Could you check a few things on this model? Use its own coordinates, in mm. Face numbers are marked on the shaded views. Give positions to 0.01 mm unless a question says otherwise; leave off trailing zeros. Put each result on its own line as item: value.
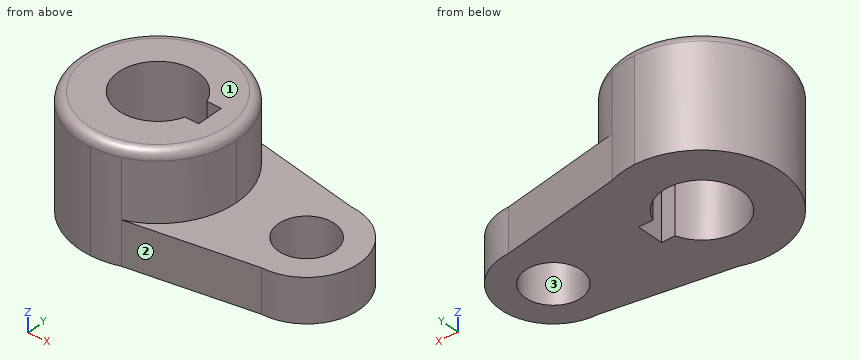
from build123d import *

# Parameters (mm, degrees)
F0_R     = 14.2875
F1_DEPTH = 40.2336
F0_R_2   = 10.16
F2_DEPTH = 15.7734
F4_DEPTH = 40.2336


# Not quite as in the source:
# - a fillet or chamfer that OpenCascade refuses, or shapes differently, is made with other operations: its cross-section is extruded or revolved along the edge and cut away or added


with BuildPart() as f1:
    # F0 (on Top) → F1 (new body)
    with BuildSketch(Plane.XY):
        with BuildLine():
            ThreePointArc((9.780704698, 26.8489932886), (4.9659159165, 28.1401901932), (0, 28.575))
            Line((0, 28.575), (9.780704698, 26.8489932886))
        make_face()
        with BuildLine():
            Line((9.780704698, -26.8489932886), (0, -28.575))
            ThreePointArc((0, -28.575), (4.9659159165, -28.1401901932), (9.780704698, -26.8489932886))
        make_face()
        with BuildLine():
            Line((9.780704698, 26.8489932886), (0, 28.575))
            ThreePointArc((0, 28.575), (-28.575, 0), (0, -28.575))
            Line((0, -28.575), (9.780704698, -26.8489932886))
            ThreePointArc((9.780704698, -26.8489932886), (23.4095521288, -16.3866864902), (28.575, 0))
            ThreePointArc((28.575, 0), (23.4095521288, 16.3866864902), (9.780704698, 26.8489932886))
        make_face()
        Circle(F0_R, mode=Mode.SUBTRACT)
    extrude(amount=F1_DEPTH)

    # F0 (on Top) → F2 (join)
    with BuildSketch(Plane.XY):
        with BuildLine():
            Line((53.975, 19.05), (9.780704698, 26.8489932886))
            ThreePointArc((9.780704698, 26.8489932886), (23.4095521288, 16.3866864902), (28.575, 0))
            ThreePointArc((28.575, 0), (23.4095521288, -16.3866864902), (9.780704698, -26.8489932886))
            Line((9.780704698, -26.8489932886), (53.975, -19.05))
            ThreePointArc((53.975, -19.05), (73.025, 0), (53.975, 19.05))
        make_face()
        with Locations((53.975, 0)):
            Circle(F0_R_2, mode=Mode.SUBTRACT)
    extrude(amount=F2_DEPTH)

    # F3 (on face) → F4 (cut, through all)
    with BuildSketch(Plane.XY.offset(40.2336)):
        with BuildLine():
            Line((18.5357414117, 5.2549776766), (13.2860026294, 5.2549776766))
            ThreePointArc((13.2860026294, 5.2549776766), (14.0348925685, 2.6747797744), (14.2875, 0))
            ThreePointArc((14.2875, 0), (14.1130788652, -2.2256821862), (13.5940741111, -4.3970223234))
            Line((13.5940741111, -4.3970223234), (18.5357414117, -4.3970223234))
            Line((18.5357414117, -4.3970223234), (18.5357414117, 5.2549776766))
        make_face()
    extrude(amount=-F4_DEPTH, mode=Mode.SUBTRACT)

    # F5: fillet of radius 3.302 on 1 edges, made by hand

    # F5_s1 → F5_t2 (revolve, cut)
    with BuildSketch(Plane.YZ):
        with BuildLine():
            ThreePointArc((28.575, 36.9316), (27.6078665915, 39.2664665915), (25.273, 40.2336))
            Line((25.273, 40.2336), (28.575, 40.2336))
            Line((28.575, 40.2336), (28.575, 36.9316))
        make_face()
    revolve(axis=Axis((0, 0, 40.2336), (0, 0, 1)), mode=Mode.SUBTRACT)


solid = f1.part
1) We'd pull the mould along X, two halves only. Please class the marked faces 1, 2 and 3: pulls with the +X half, pulls with the -X half, needs draft (parallel to the pull), parting line crosses it, or undercut.
Filled in:
face 1: needs draft
face 2: pulls with the +X half
face 3: undercut
2) If I drill on line 1 (X direction, y = 0, z = 19) (1 decimal); line 2 (X direction, y = 6.5, z = 11); line 3 (X direction, y = 7.5, z = 14.5), over which ranges is the centre line in solid material (lowest first)? Write a range as [from, to].
Filled in:
line 1: x = [-28.6, -14.3], [18.5, 28.6]
line 2: x = [-27.83, -12.72], [12.72, 46.17], [61.78, 71.88]
line 3: x = [-27.57, -12.16], [12.16, 47.12], [60.83, 71.49]
3) Suppose I cut it at A-A, the plane z = 11.5. State how many separate pieces and enclosed holes the cut face has, and give its area (3 significant figures).
Filled in:
separate pieces: 1
enclosed holes: 2
area: 3,420 mm^2
4) I'm going to push flat-ended pins straight in: pin 1 (7.5 mm diameter, centred on y = 3, z = 28, fed in from -X) (3 decimals); pin 2 (6 mm diameter, centred on x = 14.5, y = 22, fed in from -Z); pin 3 (4 mm diameter, centred on x = 15.5, y = 2, fed in from -Z) (3 decimals); pin 4 (12 mm diameter, centred on y = 18, z = 8, fed in from +X). Where does each tip first touch, or does it pass through?
Filled in:
pin 1: stops at x = -28.575
pin 2: stops at z = 0
pin 3: passes through
pin 4: stops at x = 68.77
